Geometry: final body of the model. Coordinates: model frame, mm. A direction names the side the tool comes from. Coordinates: 2 decimals unless noted, no trailing zeros. Loops run counter-clockwise (first coordinate to the right, second up) from the corner with the lowest first, then second, coordinate; pieces in that order, holes last. Notation, with made-up numbers: (68, 6.5) - (78, 6.5) arc R21 ccw to (78, 21.5) - close; hole circle Ø10 at (60, 30.5). An arc over 180 degrees is marked (long way). Answer in a Markdown table with one row per item.
from build123d import *

# Parameters (mm, degrees)
F0_W     = 26
F0_H     = 20.5
F1_DEPTH = 12
F3_R     = 1.5
F5_D     = 1.5
F6_D     = 1.5
F7_D     = 1.5
F8_D     = 1.5
F2_W     = 10
F2_H     = 4
F9_DEPTH = 10


with BuildPart() as f1:
    # F0 (on Top) → F1 (new body)
    with BuildSketch(Plane.XY):
        with Locations((-2.261453, -1.401873)):
            Rectangle(F0_W, F0_H)
        Polygon((-11.761453, -10.151873), (-11.761453, 7.348127), (5.738547, 7.348127), (7.238547, 7.348127), (7.238547, -10.151873), (5.738547, -10.151873), align=None, mode=Mode.SUBTRACT)
    extrude(amount=F1_DEPTH)

    # F3
    f3_edges = [f1.edges().sort_by_distance(p)[0] for p in [
        (10.738547, 8.848127, 6),
        (10.738547, -11.651873, 6),
        (-15.261453, -11.651873, 6),
        (-15.261453, 8.848127, 6),
    ]]
    fillet(f3_edges, radius=F3_R)

    # F5 (through all)
    with Locations(Plane.XY.offset(12)):
        with Locations((-13.061453, 2.798127)):
            Hole(F5_D / 2)

    # F6 (through all)
    with Locations(Plane.XY.offset(12)):
        with Locations((-13.061453, -5.601873)):
            Hole(F6_D / 2)

    # F7 (through all)
    with Locations(Plane.XY.offset(12)):
        with Locations((8.538547, -5.601873)):
            Hole(F7_D / 2)

    # F8 (through all)
    with Locations(Plane.XY.offset(12)):
        with Locations((8.538547, 2.798127)):
            Hole(F8_D / 2)

    # F2 (on face) → F9 (cut)
    with BuildSketch(Plane.YZ.offset(10.738547)):
        with Locations((-1.401873, 2)):
            Rectangle(F2_W, F2_H)
    extrude(amount=-F9_DEPTH, mode=Mode.SUBTRACT)


solid = f1.part
(1) First-contact query: pin 1 Ø3 at (x, y) = (8.5, -1) entering from -Z. Flat tip, straight axial feed; report the tip coordinate or a pass-through.
Verdict:
| item | result |
|---|---|
| pin 1 | stops at z = 4 |
(2) Cut plane D-D on z = 1.25. Output: boundary loops of the cut face in (x, y), then the cut area to 3 significant figures.
Verdict:
| item | result |
|---|---|
| outline | (-15.26, -10.15) arc R1.5 ccw to (-13.76, -11.65) - (9.24, -11.65) arc R1.5 ccw to (10.74, -10.15) - (10.74, -6.4) - (7.24, -6.4) - (7.24, -10.15) - (-11.76, -10.15) - (-11.76, 7.35) - (7.24, 7.35) - (7.24, 3.6) - (10.74, 3.6) - (10.74, 7.35) arc R1.5 ccw to (9.24, 8.85) - (-13.76, 8.85) arc R1.5 ccw to (-15.26, 7.35) - close; hole circle Ø1.5 at (-13.06, -5.6); hole circle Ø1.5 at (-13.06, 2.8) |
| area | 160 mm² |
(3) Cut plane C-C on z = 6. Output: boundary loops of the cut face in (x, y).
Verdict:
| item | result |
|---|---|
| outline | (-15.26, -10.15) arc R1.5 ccw to (-13.76, -11.65) - (9.24, -11.65) arc R1.5 ccw to (10.74, -10.15) - (10.74, 7.35) arc R1.5 ccw to (9.24, 8.85) - (-13.76, 8.85) arc R1.5 ccw to (-15.26, 7.35) - close; hole circle Ø1.5 at (-13.06, -5.6); hole circle Ø1.5 at (-13.06, 2.8); hole (-11.76, -10.15) - (7.24, -10.15) - (7.24, 7.35) - (-11.76, 7.35) - close; hole circle Ø1.5 at (8.54, -5.6); hole circle Ø1.5 at (8.54, 2.8) |
(4) Ray query, probe 1 along X at (y, z) = (-5.5, 11.75); probe 2 along Y at (x, z) = (2.5, 6.5); probe 3 along X at (y, z) = (-9, 0.5). Return the intervals inside material, ascending.
Verdict:
| item | result |
|---|---|
| probe 1 | x = -15.26 to -13.8, -12.32 to -11.76, 7.24 to 7.8, 9.28 to 10.74 |
| probe 2 | y = -11.65 to -10.15, 7.35 to 8.85 |
| probe 3 | x = -15.26 to -11.76, 7.24 to 10.74 |
(5) Access query for faces 1 (the face through (-2, 7.348, 6)), 2 (the face through (10.739, -2, 7)), 3 (the face through (9, -1, 4)). Directions: +Z, -Z, +X, -X, +Y, -Y. A direction counts if a zero-diameter tool reaches every point of the face in a straight line with its end or side. Return the directions, or none.
Verdict:
| item | result |
|---|---|
| face 1 | +Z, -Z |
| face 2 | +Z, -Z, +X, +Y, -Y |
| face 3 | -Z, +X |
(6) Cut plane B-B on x = 4.5. Output: boundary loops of the cut face in (y, z).
Verdict:
| item | result |
|---|---|
| outline | (-11.65, 0) - (-10.15, 0) - (-10.15, 12) - (-11.65, 12) - close; (7.35, 0) - (8.85, 0) - (8.85, 12) - (7.35, 12) - close |
(7) Cut plane A-A on y = 5.25. Output: boundary loops of the cut face in (x, z), then the cut area to 3 significant figures.
Verdict:
| item | result |
|---|---|
| outline | (-15.26, 0) - (-11.76, 0) - (-11.76, 12) - (-15.26, 12) - close; (7.24, 0) - (10.74, 0) - (10.74, 12) - (7.24, 12) - close |
| area | 84.0 mm² |
